Autodesk Inventor part; units mm, degrees
ref_plane "РабПлоскость2" through (-5.9972, 7.2, -2.1597) normal (0, 0, 1) x (1, 0, 0)
ref_plane "YZ Plane" through (0, 0, 0) normal (1, 0, 0) x (0, 1, 0)
ref_plane "XZ Plane" through (0, 0, 0) normal (0, 1, 0) x (-1, 0, 0)
sketch "Эскиз1" plane through (0, 0, 0) normal (0, 0, 1) x (1, 0, 0)
  line L0 (-4.25, 4.25) -> (4.25, 4.25)
  line L1 (4.25, 4.25) -> (4.25, -4.25)
  line L2 (4.25, -4.25) -> (-4.25, -4.25)
  line L3 (-4.25, -4.25) -> (-4.25, 4.25)
  line L4 (7, -7) -> (7, 7)
  line L5 (-7, 7) -> (-7, 4.25)
  line L6 (-7, 4.25) -> (-11, 4.25)
  line L7 (-11, 4.25) -> (-11, -4.25)
  line L8 (-11, -4.25) -> (-7, -4.25)
  line L9 (-7, -4.25) -> (-7, -7)
  line L10 (-3.75, 3.75) -> (3.75, 3.75)
  line L11 (3.75, 3.75) -> (3.75, -3.75)
  line L12 (3.75, -3.75) -> (-3.75, -3.75)
  line L13 (-3.75, -3.75) -> (-3.75, 3.75)
  line L14 (5.9972, -12) -> (5.9972, -7.2)
  line L15 (-5.9972, -7.2) -> (-5.9972, -12)
  line L16 (5.9972, -12) -> (-5.9972, -12)
  line L17 (5.9972, 7.2) -> (5.9972, 12)
  line L18 (-5.9972, 12) -> (5.9972, 12)
  line L19 (-5.9972, 12) -> (-5.9972, 7.2)
  line L20 (-5.9972, -12) -> (5.9972, -12)
  line L21 (5.9972, -12) -> (5.9972, 12)
  line L22 (5.9972, 12) -> (-5.9972, 12)
  line L23 (-5.9972, 12) -> (-5.9972, -12)
  circle A0 centre (0, -8.25) radius 1.6
  circle A1 centre (0, 8.25) radius 1.6
  point P0 (0, 0)
  dimension "d0" = 0.5
extrude "Выдавливание1" add sketch "Эскиз1" along normal blind 0.4 contours L0 L1 L2 L3 | L16 L15 L23 L19 L18 L17 L21 L14
sketch "Эскиз3" plane through (0, 0, 0) normal (0, 0, -1) x (-1, 0, 0)
  line L0 (-5.9972, 12) -> (5.9972, 12)
  line L1 (-5.9972, -12) -> (-5.9972, 12)
  line L2 (5.9972, -12) -> (-5.9972, -12)
  line L3 (5.9972, 12) -> (5.9972, -12)
  line L4 (3.75, 3.75) -> (-3.75, 3.75)
  line L5 (3.75, -3.75) -> (3.75, 3.75)
  line L6 (-3.75, -3.75) -> (3.75, -3.75)
  line L7 (-3.75, 3.75) -> (-3.75, -3.75)
  line L8 (-4.25, 4.25) -> (4.25, 4.25)
  line L9 (4.25, 4.25) -> (4.25, -4.25)
  line L10 (4.25, -4.25) -> (-4.25, -4.25)
  line L11 (-4.25, -4.25) -> (-4.25, 4.25)
  line L12 (4.5, 4.5) -> (-4.5, 4.5)
  line L13 (-4.5, 4.5) -> (-4.5, -4.5)
  line L14 (-4.5, -4.5) -> (4.5, -4.5)
  line L15 (4.5, -4.5) -> (4.5, 4.5)
  circle A0 centre (0, -8.25) radius 1.6
  circle A1 centre (0, 8.25) radius 1.6
  point P0 (0, 0)
  dimension "d6" = 0.5
  dimension "d7" = 0.25
ref_plane "РабПлоскость2" through (-5.9972, 7.2, -2.1597) normal (0, 0, 1) x (1, 0, 0)
extrude "Выдавливание3" add sketch "Эскиз3" along normal up to surface (2.1597 mm away) contours L0 L3 L2 L1
sketch "Эскиз5" plane through (5.9972, -12, -2.1597) normal (0, 0, -1) x (-1, 0, 0)
  line L0 (-1.6742, 4.8) -> (-1.6742, 19.2)
  line L1 (-1.6742, 19.2) -> (13.6686, 19.2)
  line L2 (13.6686, 19.2) -> (13.6686, 4.8)
  line L3 (13.6686, 4.8) -> (-1.6742, 4.8)
  line L4 (13.4686, 19) -> (-1.4742, 19)
  line L5 (-1.4742, 19) -> (-1.4742, 5)
  line L6 (-1.4742, 5) -> (13.4686, 5)
  line L7 (13.4686, 5) -> (13.4686, 19)
  line L8 (1.4972, 16.5) -> (10.4972, 16.5)
  line L9 (10.4972, 16.5) -> (10.4972, 7.5)
  line L10 (10.4972, 7.5) -> (1.4972, 7.5)
  line L11 (1.4972, 7.5) -> (1.4972, 16.5)
  line L12 (0, 24) -> (0, 0)
  line L13 (0, 0) -> (11.9944, 0)
  line L14 (11.9944, 0) -> (11.9944, 24)
  line L15 (11.9944, 24) -> (0, 24)
  line L16 (0, 7.5) -> (11.9944, 7.5)
  line L17 (11.9944, 16.5) -> (0, 16.5)
  line L18 (0, 7.7) -> (11.9944, 7.7)
  line L19 (11.9944, 16.3) -> (0, 16.3)
  point P0 (5.9972, 12)
  point P1 (11.9944, 5)
  point P2 (11.9944, 19)
  point P3 (0, 19)
  point P4 (0, 5)
  point P5 (10.4972, 16.3)
  point P6 (10.4972, 7.7)
  point P7 (11.9944, 7.7)
  point P8 (1.4972, 16.3)
  point P9 (0, 16.3)
  point P10 (0, 7.7)
  point P11 (1.4972, 7.7)
  dimension "d13" = 0.2
  dimension "d20" = 0.2
  dimension "d21" = 0.2
extrude "Выдавливание5" add sketch "Эскиз5" along normal blind 2 contours L12 L19 L11 L18 | L18 L9 L19 L14
sketch "Эскиз6" plane through (-5.9972, -12, 0.4) normal (0, -1, 0) x (1, 0, 0)
  line L0 (13.5091, -5.808) -> (11.9944, -2.5597)
  line L1 (11.9944, -2.5597) -> (0, -2.5597)
  line L2 (0, -2.5597) -> (-1.5147, -5.808)
  arc A0 (-1.5147, -5.808) -> (13.5091, -5.808) centre (5.9972, 3.55) ccw
  line L3 (0, -2.5597) -> (11.9944, -2.5597)
  line L4 (0, -2.5597) -> (1.1936, 0)
  line L5 (0, 0) -> (11.9944, 0)
  line L6 (11.9944, -2.5597) -> (11.9944, 0)
  line L7 (11.9944, -2.5597) -> (10.8008, 0)
  line L8 (13.4686, -2.5597) -> (11.9944, -2.5597)
  line L9 (6.996, -2.5597) -> (11.9944, -2.5597)
  line L10 (0, -2.5597) -> (-1.4742, -2.5597)
  line L11 (-1.4742, -2.5597) -> (-1.4742, -4.5597)
  line L12 (13.4686, -4.5597) -> (-1.4742, -4.5597)
  line L13 (13.4686, -2.5597) -> (13.4686, -4.5597)
  line L14 (11.9944, -2.5597) -> (11.9944, 0)
  line L15 (0, 0) -> (11.9944, 0)
  line L16 (0, -2.5597) -> (0, 0)
  line L17 (11.9944, -2.5597) -> (0, -2.5597)
  line L18 (6.996, -2.5597) -> (4.9985, -2.5597)
  line L19 (0, -2.5597) -> (4.9985, -2.5597)
  point P0 (5.9972, -0.4)
  point P1 (11.9944, -2.5597)
  point P2 (11.9944, -2.5597)
  point P3 (12.927, -4.5597)
  point P4 (-0.9326, -4.5597)
  point P5 (0, -2.5597)
  point P6 (0, -2.5597)
  point P7 (0, -2.5597)
  point P8 (0, -2.5597)
extrude "Выдавливание6" cut sketch "Эскиз6" against normal up to surface (24 mm away) contours L0 L8 L13 L12 | L7 L5 L6 | L12 L11 L10 L2 | L16 L5 L4
fillet "Сопряжение2" radius 2 2 edges at (-4.8036, 0, 0.4) (4.8036, 0, 0.4)
fillet "Сопряжение3" radius 1 10 edges at (0, -12, 0.4) (4.6041, -12, 0.0868) (5.6696, -12, -1.4572) (-5.6696, -12, -1.4572) (-4.6041, -12, 0.0868) (-5.6696, 12, -1.4572) (0, 12, 0.4) (4.6041, 12, 0.0868) (5.6696, 12, -1.4572) (-4.6041, 12, 0.0868)
chamfer "Фаска1" distance 1.5 angle 45 2 edges at (-1.6, -8.25, 0.4) (-1.6, 8.25, 0.4)
properties part number "camera_cup"
Input: part model. Units: mm. Frame: model coordinates. A direction names the side the tool comes from. Coordinates: 2 decimals unless noted, no trailing zeros. Loops run counter-clockwise (first coordinate to the right, second up) from the corner with the lowest first, then second, coordinate; pieces in that order, holes last. Notation, with made-up numbers: (-22.75, 55) - (31.25, 55) arc R21 cw to (31.25, 85) - close; hole circle Ø4 at (49, -9). An arc over 180 degrees is marked (long way). Answer in a Markdown table with one row per item. Add a question column.
Item 1: Section query B-B on y = 8.25. Return the cut outline in (x, z).
Item 2: Section query A-A on z = -2.65. Return the cut outline in (x, y).
Item 3: Access query for faces 5 (the flat face through (0, -12, -1)), 6 (the flat face through (-5, -4.3, -3)), 7 (the flat face through (-5, 4.3, -3)). Directions: +Z, -Z, +X, -X, +Y, -Y. A direction counts if a zero-diameter tool reaches every point of the face in a straight line with its end or side. Return the directions, or none.
Item 4: Mould query, pull axis X, two halves, no side actions, for faces 1 (the cylindrical face through (4.82, -0.15, -0.07)), 2 (the cylindrical face through (-5.402, -11.715, -1.594)), 3 (the cylindrical face through (0.35, 9.81, -1.62)), 4 (the flat face through (0, -4.5, -1)). Classes: released by +X, released by -X, zero draft, split by the parting line, or undercut.
Item 5: Contact query for flat-ended pins moving along their axis: P1, Ø4, axis at x = 2.5, y = 9, coming from the -Z side; P2, Ø5, axis at x = 0, y = -8.25, coming from the +Z side; P3, Ø1.5, axis at y = -7, z = -1, coming from the +X side. Output: stop coordinate, or through.
Item 6: Section query C-C on x = 0. Return the cut outline in (y, z), then the cut area to 3 significant figures.
Item 7: Section query D-D on z = -1.6. State how many separate pieces and enclosed holes the cut face has, then the cut area to 3 significant figures.
Item 8: Line query: line 1 along Y through (x, z) = (0, -1.7); line 2 along Y through (x, z) = (-1.75, -1.6); line 3 along X through (y, z) = (0.25, -2.85). Output: solid intervals per line, ascending. Write a range as [from, to].
Recorded:
| question | item | result |
|---|---|---|
| 1 | outline | (-6, -2.16) - (-1.6, -2.16) - (-1.6, -1.1) - (-3.1, 0.4) - (-3.53, 0.4) arc R2 ccw to (-5.34, -0.75) - close; (1.6, -2.16) - (6, -2.16) - (5.34, -0.75) arc R2 ccw to (3.53, 0.4) - (3.1, 0.4) - (1.6, -1.1) - close |
| 2 | outline | (-6, -4.3) - (-4.5, -4.3) - (-4.5, 4.3) - (-6, 4.3) - close; (4.5, -4.3) - (6, -4.3) - (6, 4.3) - (4.5, 4.3) - close |
| 3 | face 5 | +Z, -Z, +X, -X, -Y |
| 3 | face 6 | -Z, +X, -X, -Y |
| 3 | face 7 | -Z, +X, -X, +Y |
| 4 | face 1 | released by +X |
| 4 | face 2 | released by -X |
| 4 | face 3 | undercut |
| 4 | face 4 | undercut |
| 5 | P1 | z = -2.16 |
| 5 | P2 | z = -0.2 |
| 5 | P3 | x = 5.81 |
| 6 | outline | (-12, -2.16) - (-9.85, -2.16) - (-9.85, -1.1) - (-11.3, 0.35) arc R1 ccw to (-12, -0.6) - close; (-6.65, -2.16) - (-4.5, -2.16) - (-4.5, 0) - (-3.75, 0) - (-3.75, 0.4) - (-5.15, 0.4) - (-6.65, -1.1) - close; (3.75, 0) - (4.5, 0) - (4.5, -2.16) - (6.65, -2.16) - (6.65, -1.1) - (5.15, 0.4) - (3.75, 0.4) - close; (9.85, -2.16) - (12, -2.16) - (12, -0.6) arc R1 ccw to (11.3, 0.35) - (9.85, -1.1) - close |
| 6 | area | 17.7 mm^2 |
| 7 | separate pieces | 1 |
| 7 | enclosed holes | 3 |
| 7 | area | 177 mm^2 |
| 8 | line 1 | [-12, -9.85], [-6.65, -4.5], [4.5, 6.65], [9.85, 12] |
| 8 | line 2 | [-12, -4.5], [4.5, 12] |
| 8 | line 3 | [-6, -4.5], [4.5, 6] |
